Can you work these out from the model? Positions are in its coordinate system, mm. A direction names the side the tool comes from. Give positions to 0.01 mm unless a question says otherwise; leave off trailing zeros. Order: outer loops, then holes, each group sorted by start corner. A loop starts at its lowest first (then second) coordinate and runs counter-clockwise, first axis right, second up. Notation, with made-up numbers: (80, 34) - (98, 34) arc R23 cw to (98, 63) - close; hole circle Ø2 at (-12.75, 45.5). An arc over 180 degrees is marked (long way). Use one line per item in the form item = value. Start each with the question number.
1) Which directions (+Z, -Z, +X, -X, +Y, -Y) give clear straight access to the entire face, cutting with the end or side of a thin tool? Please do faces 1 (the flat face through (8624.29, 2954.55, 1.63)), 2 (the flat face through (8721, 2950.125, 2)), 3 (the flat face through (8744, 2935.574, 2)).
2) Suppose I cut it at A-A, the plane y = 2940. Write out the boundary of the cut face in (x, z), and give its area (3 significant figures).
3) Suppose I cut it at D-D, the plane y = 2948. Write out the boundary of the cut face in (x, z), and give its area (3 significant figures).
4) We'd pull the mould along X, two halves only. Please class faces 4 (the flat face through (8597.785, 2952, 2)), 5 (the flat face through (8624.328, 2958.845, 1.628)), 6 (the flat face through (8750.185, 2952, 2)): released by +X, released by -X, zero draft, split by the parting line, or undercut.
5) Suppose I cut it at C-C, the plane x = 8725. Write out the boundary of the cut face in (y, z).
6) For pin 1 (8 mm diameter, centred on x = 8707, y = 2954.5, fed in from -Z), with a flat end and sliding along its axis, tell me the tip position at first contact or that it passes through.
7) Suppose I cut it at B-B, the plane z = 1.3. Write out the boundary of the cut face in (x, y), and give its area (3 significant figures).
8) Please list where these lines run through material, in increasing order: probe 1 along X at (y, z) = (2939.5, 0.95); probe 2 along X at (y, z) = (2953.5, 2.95); probe 3 along Y at (x, z) = (8689.5, 1.65).
```python
from build123d import *

# Parameters (mm, degrees)
BOSS_EXTRUDE1_DEPTH = 3.302


with BuildPart() as part:
    # Sketch1 → Boss-Extrude1 (new body)
    with BuildSketch(Plane.XY):
        with BuildLine():
            Line((8750.18528935, 2968.413177756), (8597.78528935, 2968.413177756))
            Line((8597.78528935, 2968.413177756), (8597.78528935, 2935.573517756))
            Line((8597.78528935, 2935.573517756), (8629.53528935, 2935.573517756))
            Line((8629.53528935, 2935.573517756), (8629.53528935, 2943.775177756))
            ThreePointArc((8629.53528935, 2943.775177756), (8631.39516129, 2948.265305817), (8635.88528935, 2950.125177756))
            Line((8635.88528935, 2950.125177756), (8667.95278935, 2950.125177756))
            ThreePointArc((8667.95278935, 2950.125177756), (8672.442917411, 2948.265305817), (8674.30278935, 2943.775177756))
            Line((8674.30278935, 2943.775177756), (8674.30278935, 2935.573517756))
            Line((8674.30278935, 2935.573517756), (8705.41778935, 2935.573517756))
            Line((8705.41778935, 2935.573517756), (8705.41778935, 2943.775177756))
            ThreePointArc((8705.41778935, 2943.775177756), (8707.27766129, 2948.265305817), (8711.76778935, 2950.125177756))
            Line((8711.76778935, 2950.125177756), (8731.13528935, 2950.125177756))
            ThreePointArc((8731.13528935, 2950.125177756), (8735.625417411, 2948.265305817), (8737.48528935, 2943.775177756))
            Line((8737.48528935, 2943.775177756), (8737.48528935, 2935.573517756))
            Line((8737.48528935, 2935.573517756), (8750.18528935, 2935.573517756))
            Line((8750.18528935, 2935.573517756), (8750.18528935, 2968.413177756))
        make_face()
        Polygon((8618.114658264, 2961.021777756), (8615.636324499, 2956.729177756), (8618.114658264, 2952.436577756), (8623.071325795, 2952.436577756), (8625.549659561, 2956.729177756), (8623.071325795, 2961.021777756), align=None, mode=Mode.SUBTRACT)
        Polygon((8687.381955585, 2961.021777756), (8684.903621819, 2956.729177756), (8687.381955585, 2952.436577756), (8692.338623116, 2952.436577756), (8694.816956881, 2956.729177756), (8692.338623116, 2961.021777756), align=None, mode=Mode.SUBTRACT)
    extrude(amount=BOSS_EXTRUDE1_DEPTH)


solid = part.part
```
Result sheet:
q1.face_1 = +Z, -Z
q1.face_2 = +Z, -Z, -Y
q1.face_3 = +Z, -Z, +X, -X, -Y
q2.outline = (8597.79, 0) - (8629.54, 0) - (8629.54, 3.3) - (8597.79, 3.3) - close; (8674.3, 0) - (8705.42, 0) - (8705.42, 3.3) - (8674.3, 3.3) - close; (8737.49, 0) - (8750.19, 0) - (8750.19, 3.3) - (8737.49, 3.3) - close
q2.area = 250 mm²
q3.outline = (8597.79, 0) - (8631.14, 0) - (8631.14, 3.3) - (8597.79, 3.3) - close; (8672.69, 0) - (8707.03, 0) - (8707.03, 3.3) - (8672.69, 3.3) - close; (8735.88, 0) - (8750.19, 0) - (8750.19, 3.3) - (8735.88, 3.3) - close
q3.area = 271 mm²
q4.face_4 = released by -X
q4.face_5 = undercut
q4.face_6 = released by +X
q5.outline = (2950.13, 0) - (2968.41, 0) - (2968.41, 3.3) - (2950.13, 3.3) - close
q6.pin_1 = 0
q7.outline = (8597.79, 2935.57) - (8629.54, 2935.57) - (8629.54, 2943.78) arc R6.35 cw to (8635.89, 2950.13) - (8667.95, 2950.13) arc R6.35 cw to (8674.3, 2943.78) - (8674.3, 2935.57) - (8705.42, 2935.57) - (8705.42, 2943.78) arc R6.35 cw to (8711.77, 2950.13) - (8731.14, 2950.13) arc R6.35 cw to (8737.49, 2943.78) - (8737.49, 2935.57) - (8750.19, 2935.57) - (8750.19, 2968.41) - (8597.79, 2968.41) - close; hole (8615.64, 2956.73) - (8618.11, 2952.44) - (8623.07, 2952.44) - (8625.55, 2956.73) - (8623.07, 2961.02) - (8618.11, 2961.02) - close; hole (8684.9, 2956.73) - (8687.38, 2952.44) - (8692.34, 2952.44) - (8694.82, 2956.73) - (8692.34, 2961.02) - (8687.38, 2961.02) - close
q7.area = 3,790 mm²
q8.probe_1 = 8597.79 to 8629.54, 8674.3 to 8705.42, 8737.49 to 8750.19
q8.probe_2 = 8597.79 to 8617.5, 8623.69 to 8686.77, 8692.95 to 8750.19
q8.probe_3 = 2935.57 to 2952.44, 2961.02 to 2968.41
